Input: part model. Units: mm. Frame: model coordinates. A direction names the side the tool comes from. Coordinates: 2 decimals unless noted, no trailing zeros. Write each loop counter-clockwise with the first axis right and the second up, starting at its lowest first coordinate (ties: lowest second). Pieces come first, ordered by that corner, then holes. Notation, with made-up numbers: (71.25, 43.5) - (113.25, 43.5) arc R26 ccw to (113.25, 70.5) - close; hole circle Ø8 at (-20, -32.5). An arc over 180 degrees is marked (long way). Use a Markdown table: item, result. Add a question column.
Q1. Material intervals for probe 1 along Y at (x, z) = (-7.5, 2.35) (3 decimals); probe 2 along X at (y, z) = (-67.5, 0.8); probe 3 along Y at (x, z) = (5.5, 1.45) (3 decimals), sorted ascending. Write a range as from..to.
Q2. Section query C-C (z = 1.1). Give the number of separate pieces and of enclosed holes in the cut face, then the cut area to 3 significant figures.
Q3. Mould query, pull axis X, two halves, no side actions, for faces 4 (the face through (-6.094, 0.268, 1.565)), 5 (the face through (-11.45, -11.7, 1.61)), 6 (the face through (0.497, 15.867, 1.565)). Classes: released by +X, released by -X, zero draft, split by the parting line, or undercut.
Q4. Section query D-D (y = -20.5). Return the cut outline in (x, z) (1 decimal).
Q5. Section query A-A (y = 0). Return the cut outline in (x, z) (3 decimals), then the cut area to 3 significant figures.
Q6. Set-up query: faces 1 (the face through (11.112, -44, 2)), 2 (the face through (-8.129, -57.277, 1.61)), 3 (the face through (-11.112, -43, 2)). Return all of +Z, -Z, +X, -X, +Y, -Y with unobstructed straight access to the full face (end or side cutting, diameter ignored); none if empty.
Q7. Pin query (flat end, axial travel): P1, Ø5.5, axis at x = -11, y = 0, coming from the -Z side; P2, Ø1.6, axis at y = -55.5, z = 2, coming from the +X side; P3, Ø1, axis at y = -49.5, z = 1.5, coming from the -X side. Return the tip coordinate at first contact, or that it passes through.
Q8. Section query B-B (x = 0). Return the cut outline in (y, z) (3 decimals), then the cut area to 3 significant figures.
from build123d import *

# Parameters (mm, degrees)
SKETCH1_R                 = 1.65
SKETCH1_R_2               = 6.1
BOSS_EXTRUDE1_DEPTH       = 3.175
F_4_CLEARANCE_HOLE2_D     = 2.9464
F_4_CLEARANCE_HOLE2_DEPTH = 9.906
F_4_CLEARANCE_HOLE2_TIP   = 0.885187864
F_4_CLEARANCE_HOLE1_D     = 2.9464
FILLET1_R                 = 6.35


with BuildPart() as part:
    # Sketch1 → Boss-Extrude1 (new body)
    with BuildSketch(Plane.XY):
        with BuildLine():
            Line((-11.1125, -11.33701763), (-11.1125, -73.025))
            Line((-11.1125, -73.025), (11.1125, -73.025))
            Line((11.1125, -73.025), (11.1125, -11.33701763))
            ThreePointArc((11.1125, -11.33701763), (0, 15.875), (-11.1125, -11.33701763))
        make_face()
        with Locations((-11, 0)):
            Circle(SKETCH1_R, mode=Mode.SUBTRACT)
        with Locations((5.5, 9.526279442)):
            Circle(SKETCH1_R, mode=Mode.SUBTRACT)
        with Locations((5.5, -9.526279442)):
            Circle(SKETCH1_R, mode=Mode.SUBTRACT)
        Circle(SKETCH1_R_2, mode=Mode.SUBTRACT)
    extrude(amount=BOSS_EXTRUDE1_DEPTH)

    # #4 Clearance Hole2
    with Locations(Plane(origin=(0, 0, 0), x_dir=(-1, 0, 0), z_dir=(0, 0, -1))):
        with Locations((7.9375, -68.2625), (-7.9375, -68.2625), (-7.9375, -58.7375), (7.9375, -58.7375)):
            Hole(F_4_CLEARANCE_HOLE2_D / 2, depth=F_4_CLEARANCE_HOLE2_DEPTH)
            with Locations((0, 0, -(F_4_CLEARANCE_HOLE2_DEPTH + F_4_CLEARANCE_HOLE2_TIP / 2))):  # 118° drill point
                Cone(0, F_4_CLEARANCE_HOLE2_D / 2, F_4_CLEARANCE_HOLE2_TIP, mode=Mode.SUBTRACT)

    # #4 Clearance Hole1 (through all)
    with Locations(Plane(origin=(0, 0, 0), x_dir=(-1, 0, 0), z_dir=(0, 0, -1))):
        with Locations((0, -68.2625), (0, -32.7025)):
            Hole(F_4_CLEARANCE_HOLE1_D / 2)

    # Fillet1
    fillet1_edges = [part.edges().sort_by_distance(p)[0] for p in [
        (11.1125, -11.33701763, 1.5875),
        (-11.1125, -11.33701763, 1.5875),
    ]]
    fillet(fillet1_edges, radius=FILLET1_R)


solid = part.part
Values follow:
| question | item | result |
|---|---|---|
| 1 | probe 1 | -73.025..-69.669, -66.856..-60.144, -57.331..13.992 |
| 1 | probe 2 | -11.11..-9.2, -6.68..-1.26, 1.26..6.68, 9.2..11.11 |
| 1 | probe 3 | -73.025..-11.176, -7.876..-2.638, 2.638..7.876, 11.176..14.892 |
| 2 | separate pieces | 1 |
| 2 | enclosed holes | 10 |
| 2 | area | 1,910 mm2 |
| 3 | face 4 | undercut |
| 3 | face 5 | released by -X |
| 3 | face 6 | split by the parting line |
| 4 | outline | (-11.1, 0) - (11.1, 0) - (11.1, 3.2) - (-11.1, 3.2) - close |
| 5 | outline | (-15.875, 0) - (-12.65, 0) - (-12.65, 3.175) - (-15.875, 3.175) - close; (-9.35, 0) - (-6.1, 0) - (-6.1, 3.175) - (-9.35, 3.175) - close; (6.1, 0) - (15.875, 0) - (15.875, 3.175) - (6.1, 3.175) - close |
| 5 | area | 51.6 mm2 |
| 6 | face 1 | +Z, -Z, +X, -Y |
| 6 | face 2 | +Z, -Z |
| 6 | face 3 | +Z, -Z, -X, -Y |
| 7 | P1 | z = 0 |
| 7 | P2 | x = 11.11 |
| 7 | P3 | x = -11.11 |
| 8 | outline | (-73.025, 0) - (-69.736, 0) - (-69.736, 3.175) - (-73.025, 3.175) - close; (-66.789, 0) - (-34.176, 0) - (-34.176, 3.175) - (-66.789, 3.175) - close; (-31.229, 0) - (-6.1, 0) - (-6.1, 3.175) - (-31.229, 3.175) - close; (6.1, 0) - (15.875, 0) - (15.875, 3.175) - (6.1, 3.175) - close |
| 8 | area | 225 mm2 |
